Here's how the part is built. I have some questions about the finished solid (model axes, mm). A direction names the side the tool comes from. Give positions to 0.01 mm unless a question says otherwise; leave off trailing zeros. Loops run counter-clockwise (first coordinate to the right, second up) from the corner with the lowest first, then second, coordinate; pieces in that order, holes last. Notation, with made-up numbers: (56.5, 73.25) - (68.5, 73.25) arc R26 ccw to (68.5, 105.25) - close; hole circle Ø4 at (50, -13). An arc over 180 degrees is marked (long way). Return JSON: item names as keys, results as strings. Group by question number.
(1) If we section it at A-A (x = -74.5): Please give me the cut outline in (y, z), then the cut area to 3 significant figures.
(2) If we section it at D-D (x = -95.5): Please give me the cut outline in (y, z).
(3) I need wall thicknesses on probe 1 along Y at (x, z) = (-74.5, 11.5); probe 2 along Z at (x, y) = (-89.5, 15.75); probe 3 along Z at (x, y) = (-166, 14). Which ranges of each line are inside material? Lowest first, please. Write a range as [from, to].
(4) If we section it at C-C (y = 16): Please give me the cut outline in (x, z).
(5) If we mould it in two halves opening along X, with no side actions, what happens to faces 4 (the flat face through (-114, 17.792, 12)), 5 (the flat face through (-113, 9.792, 12)), 6 (the cylindrical face through (-90.174, 16.435, 5.423)), 7 (the cylindrical face through (-62.367, 16.435, 8.381))? For each: released by +X, released by -X, zero draft, split by the parting line, or undercut.
(6) For P1, Ø1.5, axis at y = 21.5, z = 5, coming from the -X side; P2, Ø5, axis at x = -132.5, y = 14, coming from the -Z side; P3, Ø1, axis at y = 15.5, z = 5.5, coming from the -X side; P4, Ø1, axis at x = -123.5, z = 9, coming from the -Y side, each with a flat end and sliding along its axis, tell me the tip position at first contact or that it passes through.
(7) If we section it at B-B (z = 2.25): Please give me the cut outline in (x, y), then the cut area to 3 significant figures.
(8) On a 3-axis mill with a long thin cutter (end or side, diameter ignored), from which of +Z, -Z, +X, -X, +Y, -Y can I reach the whole of each face in a straight line? I mean faces 1 (the flat face through (-88, 16, 11)), 2 (the flat face through (-125, 18, 17)), 3 (the cylindrical face through (-67.366, 16.325, 8.381)). Say none if no direction works.
```python
from build123d import *

# Parameters (mm, degrees)
BOSS_EXTRUDE1_DEPTH = 11
BOSS_EXTRUDE2_DEPTH = 6


with BuildPart() as part:
    # Sketch1 → Boss-Extrude1 (new body)
    with BuildSketch(Plane.XY):
        with BuildLine():
            Line((-68.865823893, 22.791817364), (-83.675684171, 22.791817364))
            ThreePointArc((-83.675684171, 22.791817364), (-90.175684171, 16.291817364), (-83.675684171, 9.791817364))
            Line((-83.675684171, 9.791817364), (-68.865823893, 9.791817364))
            ThreePointArc((-68.865823893, 9.791817364), (-62.365823893, 16.291817364), (-68.865823893, 22.791817364))
        make_face()
        with BuildLine():
            Line((-68.865823893, 17.791817364), (-83.675684171, 17.791817364))
            ThreePointArc((-83.675684171, 17.791817364), (-85.175684171, 16.291817364), (-83.675684171, 14.791817364))
            Line((-83.675684171, 14.791817364), (-68.865823893, 14.791817364))
            ThreePointArc((-68.865823893, 14.791817364), (-67.365823893, 16.291817364), (-68.865823893, 17.791817364))
        make_face(mode=Mode.SUBTRACT)
    extrude(amount=BOSS_EXTRUDE1_DEPTH)

    # Sketch2 → Boss-Extrude2 (add)
    with BuildSketch(Plane.XY.offset(11)):
        with BuildLine():
            Line((-183.675684171, 22.791817364), (-83.675684171, 22.791817364))
            Line((-83.675684171, 22.791817364), (-68.865823893, 22.791817364))
            ThreePointArc((-68.865823893, 22.791817364), (-62.365823893, 16.291817364), (-68.865823893, 9.791817364))
            Line((-68.865823893, 9.791817364), (-83.675684171, 9.791817364))
            Line((-83.675684171, 9.791817364), (-183.675684171, 9.791817364))
            ThreePointArc((-183.675684171, 9.791817364), (-190.175684171, 16.291817364), (-183.675684171, 22.791817364))
        make_face()
        with BuildLine():
            Line((-183.675684171, 17.791817364), (-83.675684171, 17.791817364))
            Line((-83.675684171, 17.791817364), (-68.865823893, 17.791817364))
            ThreePointArc((-68.865823893, 17.791817364), (-67.365823893, 16.291817364), (-68.865823893, 14.791817364))
            Line((-68.865823893, 14.791817364), (-83.675684171, 14.791817364))
            Line((-83.675684171, 14.791817364), (-183.675684171, 14.791817364))
            ThreePointArc((-183.675684171, 14.791817364), (-185.175684171, 16.291817364), (-183.675684171, 17.791817364))
        make_face(mode=Mode.SUBTRACT)
    extrude(amount=BOSS_EXTRUDE2_DEPTH)


solid = part.part
```
Values:
{
 "1": {"outline": "(9.79, 0) - (14.79, 0) - (14.79, 17) - (9.79, 17) - close; (17.79, 0) - (22.79, 0) - (22.79, 17) - (17.79, 17) - close", "area": "170 mm2"},
 "2": {"outline": "(9.79, 11) - (14.79, 11) - (14.79, 17) - (9.79, 17) - close; (17.79, 11) - (22.79, 11) - (22.79, 17) - (17.79, 17) - close"},
 "3": {"probe 1": "[9.79, 14.79], [17.79, 22.79]", "probe 2": "[0, 11]", "probe 3": "[11, 17]"},
 "4": {"outline": "(-190.17, 11) - (-185.15, 11) - (-185.15, 17) - (-190.17, 17) - close; (-90.17, 0) - (-85.15, 0) - (-85.15, 11) - (-90.17, 11) - close; (-67.39, 0) - (-62.37, 0) - (-62.37, 17) - (-67.39, 17) - close"},
 "5": {"face 4": "undercut", "face 5": "zero draft", "face 6": "released by -X", "face 7": "released by +X"},
 "6": {"P1": "x = -88.41", "P2": "z = 11", "P3": "x = -90.17", "P4": "through"},
 "7": {"outline": "(-83.68, 9.79) - (-68.87, 9.79) arc R6.5 ccw to (-68.87, 22.79) - (-83.68, 22.79) arc R6.5 ccw to start; hole (-83.68, 14.79) - (-68.87, 14.79) arc R1.5 ccw to (-68.87, 17.79) - (-83.68, 17.79) arc R1.5 ccw to start", "area": "274 mm2"},
 "8": {"face 1": "+Z", "face 2": "+Z, +X, -X, +Y, -Y", "face 3": "+Z, -Z"}
}
